The figure shows three views and two pictorial views of one solid part (mm, origin at its lowest corner). Answer the questions. A direction names the side the tool comes from. Coordinates: 2 decimals unless noted, no trailing zeros. Write each loop counter-clockwise with the first axis right and the second up, starting at its lowest first coordinate (ties: lowest second). Pieces come first, ordered by that corner, then holes. Notation, with made-up numbers: M 70.5,76.25 L 96.5,76.25 A21 ccw 96.5,94.25 Z; hole C 34.25,53 d5. An arc over 180 degrees is marked long. Use a Markdown table: item, result. Add a question column.
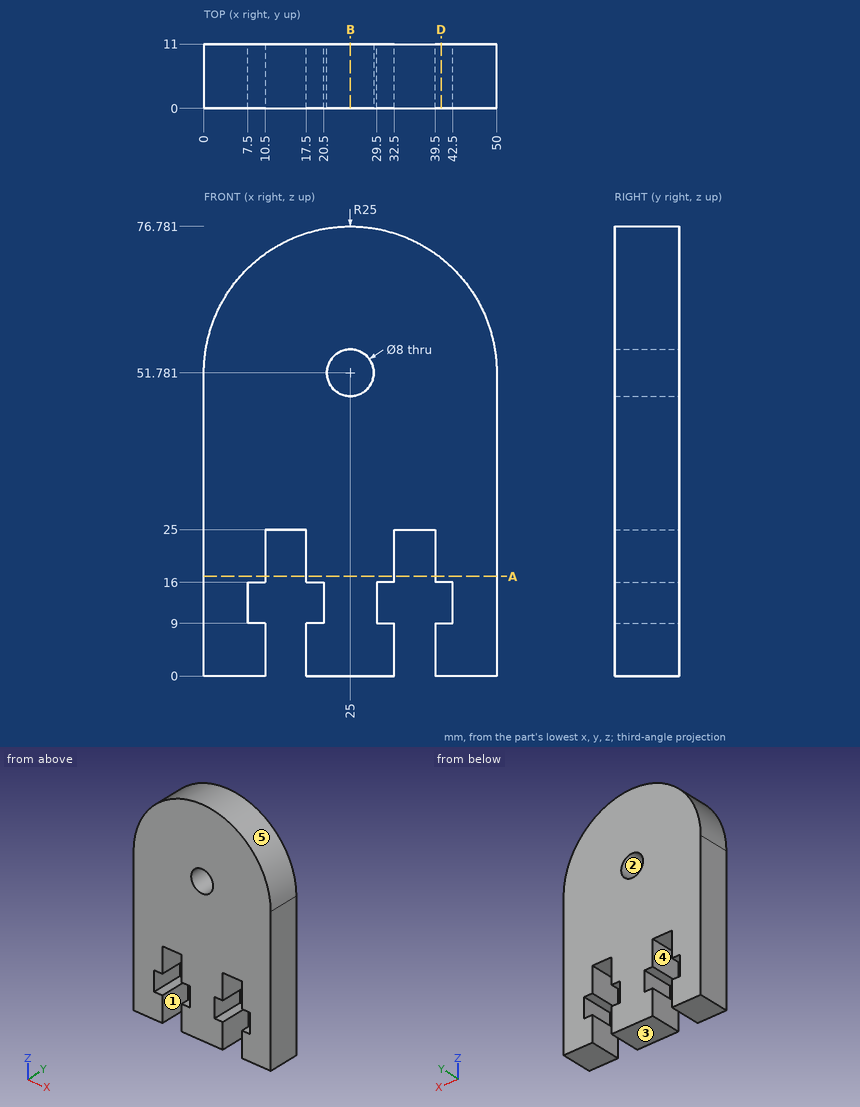
Item 1: Consider probe 1 along X at (y, z) = (10, 18.5); probe 2 along X at (y, z) = (2.75, 10.5); probe 3 along Z at (x, y) = (25, 3.75). Determine where each line is inside the solid, lowest interval first.
Item 2: For the marked faces 4 and 5, determine the directions among +Z, -Z, +X, -X, +Y, -Y from which every point of the face is accessible in a straight line to the end or side of a thin tool.
Item 3: Find section B-B on x = 25. Give the vertices of the cut face in (y, z).
Item 4: Determine the mould class of the marked faces 1, 2 and 3 for opening direction Z: pulls with the +Z half, pulls with the -Z half, needs draft (parallel to the pull), parting line crosses it, or undercut.
Item 5: Find section D-D on x = 40.5. Give the vertices of the cut face in (y, z), then the cut area to 3 significant figures.
Item 6: This flat-tipped pin is pushed along its axis until it touches: pin 1 (3.5 mm diameter, centred on x = 9, y = 5, fed in from +Z). Where does it stop, or does it pass through?
Item 7: Find section A-A on z = 17. Give the vertices of the cut face in (x, y).
Geometry says:
| question | item | result |
|---|---|---|
| 1 | probe 1 | x = 0 to 10.5, 17.5 to 32.5, 39.5 to 50 |
| 1 | probe 2 | x = 0 to 7.5, 20.5 to 29.5, 42.5 to 50 |
| 1 | probe 3 | z = 0 to 47.78, 55.78 to 76.78 |
| 2 | face 4 | -Z, +Y, -Y |
| 2 | face 5 | +Z, +Y, -Y |
| 3 | outline | M 0,0 L 11,0 L 11,47.78 L 0,47.78 Z; M 0,55.78 L 11,55.78 L 11,76.78 L 0,76.78 Z |
| 4 | face 1 | needs draft |
| 4 | face 2 | undercut |
| 4 | face 3 | pulls with the -Z half |
| 5 | outline | M 0,0 L 11,0 L 11,9 L 0,9 Z; M 0,16 L 11,16 L 11,71.4 L 0,71.4 Z |
| 5 | area | 708 mm2 |
| 6 | pin 1 | stops at z = 72.32 |
| 7 | outline | M 0,0 L 10.5,0 L 10.5,11 L 0,11 Z; M 17.5,0 L 32.5,0 L 32.5,11 L 17.5,11 Z; M 39.5,0 L 50,0 L 50,11 L 39.5,11 Z |
